Design review of the part built by this model. Coordinates are the model's own, in mm. Face numbers are marked on the shaded views. Coordinates: 2 decimals unless noted, no trailing zeros. Loops run counter-clockwise (first coordinate to the right, second up) from the corner with the lowest first, then second, coordinate; pieces in that order, holes last. Notation, with made-up numbers: (19.5, 54) -> (73.5, 54) arc R23 ccw to (73.5, 75) -> close; hole circle Ø2 at (55, -25). An arc over 180 degrees is marked (long way). Answer as a JSON object with one key per item and string values.
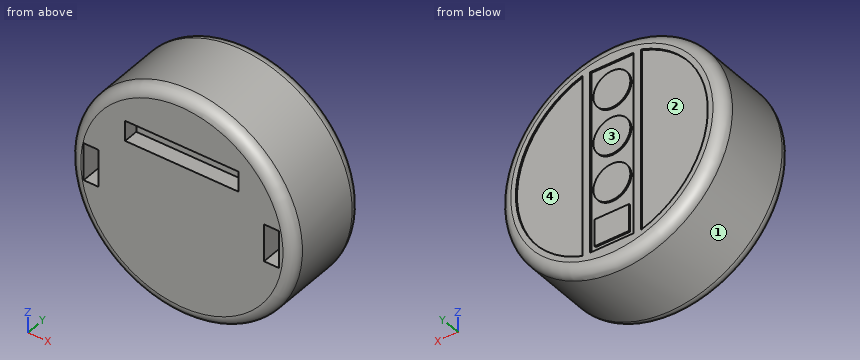
```python
from build123d import *

# Parameters (mm, degrees)
SKETCH1_R           = 190.5
BOSS_EXTRUDE1_DEPTH = 152.4
SKETCH4_W           = 73.557387936
SKETCH4_H           = 310.235544462
CUT_EXTRUDE2_DEPTH  = 2.54
SKETCH5_R           = 31.334472959
SKETCH5_W           = 58.317387936
SKETCH5_H           = 46.041460357
BOSS_EXTRUDE3_DEPTH = 2.54
SKETCH6_W           = 25.4
SKETCH6_H           = 63.5
CUT_EXTRUDE3_DEPTH  = 38.1
FILLET3_R           = 19.05
SKETCH8_W           = 192.151300236
SKETCH8_H           = 34.488694915
CUT_EXTRUDE4_DEPTH  = 25.4


with BuildPart() as part:
    # Sketch1 → Boss-Extrude1 (new body)
    with BuildSketch(Plane(origin=(0, 0, 0), x_dir=(1, 0, 0), z_dir=(0, 1, 0))):
        with Locations(Location((0, 0, 0), (0, 0, 90))):
            Circle(SKETCH1_R)
    extrude(amount=BOSS_EXTRUDE1_DEPTH)

    # Sketch4 → Cut-Extrude2 (cut)
    with BuildSketch(Plane(origin=(0, 152.4, 0), x_dir=(1, 0, 0), z_dir=(0, 1, 0))):
        with BuildLine():
            Line((-49.478693968, 155.117772231), (-49.478693968, -155.117772231))
            ThreePointArc((-49.478693968, -155.117772231), (-162.817887281, 0), (-49.478693968, 155.117772231))
        make_face()
        with BuildLine():
            Line((49.478693968, 155.117772231), (49.478693968, -155.117772231))
            ThreePointArc((49.478693968, -155.117772231), (162.817887281, 0), (49.478693968, 155.117772231))
        make_face()
        Rectangle(SKETCH4_W, SKETCH4_H)
    extrude(amount=-CUT_EXTRUDE2_DEPTH, mode=Mode.SUBTRACT)

    # Sketch5 → Boss-Extrude3 (add)
    with BuildSketch(Plane(origin=(0, 149.86, 0), x_dir=(1, 0, 0), z_dir=(0, 1, 0))):
        with Locations(Location((0, 50.250313703, 0), (0, 0, 270))):
            Circle(SKETCH5_R)
        with Locations(Location((0, -29.505686297, 0), (0, 0, 90))):
            Circle(SKETCH5_R)
        with Locations(Location((0, -109.261686297, 0), (0, 0, 90))):
            Circle(SKETCH5_R)
        with Locations((0, 124.477042052)):
            Rectangle(SKETCH5_W, SKETCH5_H)
    extrude(amount=BOSS_EXTRUDE3_DEPTH)

    # Sketch6 → Cut-Extrude3 (cut)
    with BuildSketch(Plane.XZ):
        with Locations((-153.728334256, 2.735150341)):
            Rectangle(SKETCH6_W, SKETCH6_H)
        with Locations((152.139955728, 2.262697534)):
            Rectangle(SKETCH6_W, SKETCH6_H)
    extrude(amount=-CUT_EXTRUDE3_DEPTH, mode=Mode.SUBTRACT)

    # Fillet3
    fillet3_edges = [part.edges().sort_by_distance(p)[0] for p in [
        (0, 0, 190.5),
        (0, 152.4, 190.5),
    ]]
    fillet(fillet3_edges, radius=FILLET3_R)

    # Sketch8 → Cut-Extrude4 (cut)
    with BuildSketch(Plane.XZ):
        with Locations((0, 87.69982421)):
            Rectangle(SKETCH8_W, SKETCH8_H)
    extrude(amount=-CUT_EXTRUDE4_DEPTH, mode=Mode.SUBTRACT)


solid = part.part
```
1) Add section B-B, the plane y = 87.5. Give the boundary of the cut face in (x, z).
Completed:
{"outline": "circle Ø381 at (0, 0)"}
2) Clearance check with flat-ended pins moving along their axes: pin 1 Ø7.5 at (y, z) = (7, 89) entering from -X; pin 2 Ø8 at (x, z) = (151, 28) entering from -Y; pin 3 Ø1.3 at (x, y) = (14, 150.5) entering from -Z. State where each tip first meets the part, or that it passes through.
Completed:
{"pin 1": "x = -167.03", "pin 2": "y = 38.1", "pin 3": "z = -180.43"}
3) The part is to be moulded in two halves that separate along X. For the marked faces 1, 2, 3 and 4, say which applies: pulls with the +X half, pulls with the -X half, needs draft (parallel to the pull), parting line crosses it, or undercut.
Completed:
{"face 1": "parting line crosses it", "face 2": "undercut", "face 3": "needs draft", "face 4": "undercut"}
4) Wall thickness on probe 1 along Y at (x, z) = (-157, 26); probe 2 along X at (y, z) = (11.5, 79.5); probe 3 along Y at (x, z) = (-27, 74.5): over which ranges is each line inside the solid? List them lowest first.
Completed:
{"probe 1": "38.1 to 149.86", "probe 2": "-171.4 to -96.08, 96.08 to 171.4", "probe 3": "25.4 to 149.86"}
